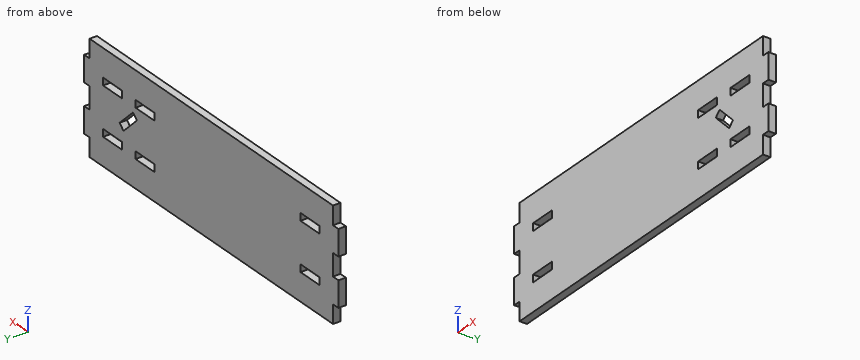
```python
from build123d import *

# Parameters (mm, degrees)
SKETCH1_W           = 2
SKETCH1_H           = 7
SKETCH1_W_2         = 7
SKETCH1_H_2         = 2
BOSS_EXTRUDE1_DEPTH = 2


with BuildPart() as part:
    # Sketch1 → Boss-Extrude1 (new body)
    # profile 1 of 6: a face of its own
    with BuildSketch(Plane(origin=(0, 0, 0), x_dir=(1, 0, 0), z_dir=(0, 1, 0))):
        with Locations((-24.050101389, 5.323848353)):
            Rectangle(SKETCH1_W, SKETCH1_H)
    # profile 2 of 6: a face of its own
    with BuildSketch(Plane(origin=(0, 0, 0), x_dir=(1, 0, 0), z_dir=(0, 1, 0))):
        with Locations((-24.050101389, -7.676151647)):
            Rectangle(SKETCH1_W, SKETCH1_H)
    # profile 3 of 6: a face of its own
    with BuildSketch(Plane(origin=(0, 0, 0), x_dir=(1, 0, 0), z_dir=(0, 1, 0))):
        Polygon((66.949898611, 13.823848353), (-23.050101389, 13.823848353), (-23.050101389, 8.823848353), (-23.050101389, 1.823848353), (-23.050101389, -4.176151647), (-23.050101389, -11.176151647), (-23.050101389, -16.176151647), (66.949898611, -16.176151647), (66.949898611, -11.176151647), (66.949898611, -4.176151647), (66.949898611, 1.823848353), (66.949898611, 8.823848353), align=None)
        with Locations((-14.550101389, -7.676151647)):
            Rectangle(SKETCH1_W_2, SKETCH1_H_2, mode=Mode.SUBTRACT)
        with Locations((46.449898611, -7.676151647)):
            Rectangle(SKETCH1_W_2, SKETCH1_H_2, mode=Mode.SUBTRACT)
        with Locations((58.449898611, -7.676151647)):
            Rectangle(SKETCH1_W_2, SKETCH1_H_2, mode=Mode.SUBTRACT)
        Polygon((54.425685048, 1.299905334), (55.839898611, -0.114308229), (50.890151142, -5.064055697), (49.47593758, -3.649842135), align=None, mode=Mode.SUBTRACT)
        with Locations((-14.550101389, 5.323848353)):
            Rectangle(SKETCH1_W_2, SKETCH1_H_2, mode=Mode.SUBTRACT)
        with Locations((46.449898611, 5.323848353)):
            Rectangle(SKETCH1_W_2, SKETCH1_H_2, mode=Mode.SUBTRACT)
        with Locations((58.449898611, 5.323848353)):
            Rectangle(SKETCH1_W_2, SKETCH1_H_2, mode=Mode.SUBTRACT)
    # profile 4 of 6: a face of its own
    with BuildSketch(Plane(origin=(0, 0, 0), x_dir=(1, 0, 0), z_dir=(0, 1, 0))):
        with Locations((67.949898611, 5.323848353)):
            Rectangle(SKETCH1_W, SKETCH1_H)
    # profile 5 of 6: a face of its own
    with BuildSketch(Plane(origin=(0, 0, 0), x_dir=(1, 0, 0), z_dir=(0, 1, 0))):
        with Locations((67.949898611, -7.676151647)):
            Rectangle(SKETCH1_W, SKETCH1_H)
    # profile 6 of 6: a face of its own
    with BuildSketch(Plane(origin=(0, 0, 0), x_dir=(1, 0, 0), z_dir=(0, 1, 0))):
        Polygon((66.949898611, 13.823848353), (-23.050101389, 13.823848353), (-23.050101389, 8.823848353), (-23.050101389, 1.823848353), (-23.050101389, -4.176151647), (-23.050101389, -11.176151647), (-23.050101389, -16.176151647), (66.949898611, -16.176151647), (66.949898611, -11.176151647), (66.949898611, -4.176151647), (66.949898611, 1.823848353), (66.949898611, 8.823848353), align=None)
        with Locations((-14.550101389, -7.676151647)):
            Rectangle(SKETCH1_W_2, SKETCH1_H_2, mode=Mode.SUBTRACT)
        with Locations((46.449898611, -7.676151647)):
            Rectangle(SKETCH1_W_2, SKETCH1_H_2, mode=Mode.SUBTRACT)
        with Locations((58.449898611, -7.676151647)):
            Rectangle(SKETCH1_W_2, SKETCH1_H_2, mode=Mode.SUBTRACT)
        Polygon((54.425685048, 1.299905334), (55.839898611, -0.114308229), (50.890151142, -5.064055697), (49.47593758, -3.649842135), align=None, mode=Mode.SUBTRACT)
        with Locations((-14.550101389, 5.323848353)):
            Rectangle(SKETCH1_W_2, SKETCH1_H_2, mode=Mode.SUBTRACT)
        with Locations((46.449898611, 5.323848353)):
            Rectangle(SKETCH1_W_2, SKETCH1_H_2, mode=Mode.SUBTRACT)
        with Locations((58.449898611, 5.323848353)):
            Rectangle(SKETCH1_W_2, SKETCH1_H_2, mode=Mode.SUBTRACT)
    extrude(amount=BOSS_EXTRUDE1_DEPTH)


solid = part.part
```
The model under review builds one solid part; all positions refer to its coordinate system, in mm. Coordinates: 2 decimals unless noted, no trailing zeros. Write each loop counter-clockwise with the first axis right and the second up, starting at its lowest first coordinate (ties: lowest second). Pieces come first, ordered by that corner, then holes.
1) We need section A-A on x = -16. State the section outline as (y, z) points, then the cut area to 3 significant figures.
2) To check wall thickness, follow probe 1 along Z at (x, y) = (48, 1.5); probe 2 along X at (y, z) = (1.7, 8.5); probe 3 along X at (y, z) = (1.4, 14.5). State the ranges of each line that lie inside material, in increasing order.
3) Clearance check with flat-ended pins moving along their axes: pin 1 Ø0.6 at (y, z) = (0.5, 14) entering from +X; pin 2 Ø0.6 at (x, y) = (-24, 0.5) entering from +Z; pin 3 Ø1 at (x, y) = (68.5, 1) entering from -Z. State where each tip first meets the part, or that it passes through.
4) We need section C-C on z = -12. State the section outline as (x, y) points, then the cut area to 3 significant figures.
5) We need section B-B on y = 1.45. Count the separate pieces of the cut face and the enclosed holes in it, then the cut area to 3 significant figures.
Answer list:
1. outline: (0, -13.82) - (2, -13.82) - (2, -6.32) - (0, -6.32) - close; (0, -4.32) - (2, -4.32) - (2, 6.68) - (0, 6.68) - close; (0, 8.68) - (2, 8.68) - (2, 16.18) - (0, 16.18) - close
1. area: 52.0 mm2
2. probe 1: z = -13.82 to -6.32, -4.32 to 6.68, 8.68 to 16.18
2. probe 2: x = -25.05 to -18.05, -11.05 to 42.95, 49.95 to 54.95, 61.95 to 68.95
2. probe 3: x = -23.05 to 66.95
3. pin 1: stops at x = 66.95
3. pin 2: stops at z = 11.18
3. pin 3: stops at z = -8.82
4. outline: (-23.05, 0) - (66.95, 0) - (66.95, 2) - (-23.05, 2) - close
4. area: 180 mm2
5. separate pieces: 1
5. enclosed holes: 7
5. area: 2,660 mm2
